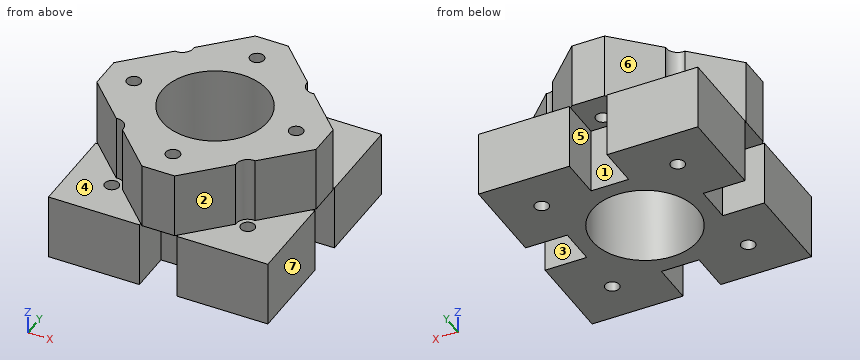
```python
from build123d import *

# Parameters (mm, degrees)
SKETCH_1_W          = 50
SKETCH_1_H          = 50
EXTRUDE_1_DEPTH     = 30
HOLE_WIZARD_348_D   = 24
HOLE_WIZARD_1_D     = 3.2
HOLE_WIZARD_2_D     = 3.2
CUT_EXTRUDE_1_DEPTH = 15
SKETCH_16_W         = 8.580132312
SKETCH_16_H         = 9.5
SKETCH_16_W_2       = 9.5
SKETCH_16_H_2       = 8.580132312
CUT_EXTRUDE_3_DEPTH = 15
HOLE_WIZARD_3_D     = 5.2
HOLE_WIZARD_3_DEPTH = 15


with BuildPart() as part:
    # 草图1 → 凸台-拉伸1 (new body)
    with BuildSketch(Plane.XY):
        Rectangle(SKETCH_1_W, SKETCH_1_H)
    extrude(amount=EXTRUDE_1_DEPTH)

    # Hole Wizard 348 (through all)
    with Locations(Plane.XY.offset(30)):
        with Locations((0, 0)):
            Hole(HOLE_WIZARD_348_D / 2)

    # 孔1 (through all)
    with Locations(Plane.XY.offset(30)):
        with Locations((-15.5, 15.5), (15.5, 15.5), (15.5, -15.5), (-15.5, -15.5)):
            Hole(HOLE_WIZARD_1_D / 2)

    # 孔2 (through all)
    with Locations(Plane.XY.offset(30)):
        with Locations((0, 18.5), (18.5, 0), (0, -18.5), (-18.5, 0)):
            Hole(HOLE_WIZARD_2_D / 2)

    # 草图13 → 切除-拉伸-薄壁1 (cut)
    with BuildSketch(Plane.XY.offset(30)):
        Polygon((-25, 3.7372583), (-14.36862915, 14.36862915), (-3.7372583, 25), (-17.879393924, 39.142135624), (-28.510764774, 28.510764774), (-39.142135624, 17.879393924), align=None)
        Polygon((3.7372583, 25), (14.36862915, 14.36862915), (25, 3.7372583), (39.142135624, 17.879393924), (28.510764774, 28.510764774), (17.879393924, 39.142135624), align=None)
        Polygon((-3.7372583, -25), (-14.36862915, -14.36862915), (-25, -3.7372583), (-39.142135624, -17.879393924), (-28.510764774, -28.510764774), (-17.879393924, -39.142135624), align=None)
        Polygon((25, -3.7372583), (14.36862915, -14.36862915), (3.7372583, -25), (17.879393924, -39.142135624), (28.510764774, -28.510764774), (39.142135624, -17.879393924), align=None)
    extrude(amount=-CUT_EXTRUDE_1_DEPTH, mode=Mode.SUBTRACT)

    # 草图16 → 切除-拉伸3 (cut)
    with BuildSketch(Plane(origin=(0, 0, 0), x_dir=(-1, 0, 0), z_dir=(0, 0, -1))):
        with Locations((0, 20.25)):
            Rectangle(SKETCH_16_W, SKETCH_16_H)
        with Locations((0, -20.25)):
            Rectangle(SKETCH_16_W, SKETCH_16_H)
        with Locations((-20.25, 0)):
            Rectangle(SKETCH_16_W_2, SKETCH_16_H_2)
        with Locations((20.25, 0)):
            Rectangle(SKETCH_16_W_2, SKETCH_16_H_2)
    extrude(amount=-CUT_EXTRUDE_3_DEPTH, mode=Mode.SUBTRACT)

    # 孔3
    with Locations(Plane.XY.offset(30)):
        with Locations((-15.5, 15.5), (15.5, 15.5), (15.5, -15.5), (-15.5, -15.5)):
            Hole(HOLE_WIZARD_3_D / 2, depth=HOLE_WIZARD_3_DEPTH)


solid = part.part
```
Check sheet for the modelled part. Datum: model origin and axes. Units: mm. Face numbers are marked on the shaded views. A direction names the side the tool comes from. Coordinates: 2 decimals unless noted, no trailing zeros. Order: outer loops, then holes, each group sorted by start corner. A loop starts at its lowest first (then second) coordinate and runs counter-clockwise, first axis right, second up. Notation, with made-up numbers: M -15,-32 L 14,-32 A37 ccw 14,7 Z; hole C 43,57 d1. An arc over 180 degrees is marked long. Write each question's results on one line, items separated by ' | '. Start each with the question number.
1. Access from +Z, -Z, +X, -X, +Y, -Y to the whole of each face (thin tool, end or side, straight path). Record for the marked faces 1, 2, 3 and 4.
2. Mould release check, pull along X, two halves, no side actions. Record for the marked faces 5, 6 and 7: +X half, -X half, draft (parallel to the pull), parting line (faces both ways), or undercut.
3. Material ranges on probe 1 along Y at (x, z) = (0, 26.25); probe 2 along X at (y, z) = (17.5, 6.25); probe 3 along Z at (x, y) = (22.5, -2.5), recorded low to high.
4. Cross-section at D-D on x = 18.5. Record the cut outline in (y, z).
5. Cross-section at A-A on x = 0. Record the cut outline in (y, z), and give its area (3 significant figures).
6. Cross-section at C-C on z = 9.25. Record the cut outline in (x, y), and give its area (3 significant figures).
7. Go/stop test with flat-tipped pins: P1, Ø9.5, axis at x = 20.5, y = -0.5, coming from the -Z side; P2, Ø5, axis at x = -15.5, y = -15.5, coming from the +Z side; P3, Ø6, axis at x = 0.5, y = 19.5, coming from the -Z side; P4, Ø1.5, axis at y = -3, z = 14, coming from the +X side. Record where each tip stops, or that it passes through.
Checks:
1) face 1: -Z, +Y | face 2: +Z, +X, -Y | face 3: -Z, +X | face 4: +Z, -X, -Y
2) face 5: undercut | face 6: -X half | face 7: +X half
3) probe 1: y = -25 to -20.1, -16.9 to -12, 12 to 16.9, 20.1 to 25 | probe 2: x = -25 to -4.29, 4.29 to 25 | probe 3: z = 15 to 30
4) outline: M -25,0 L -4.29,0 L -4.29,15 L -1.6,15 L -1.6,30 L -10.24,30 L -10.24,15 L -25,15 Z; M 1.6,15 L 4.29,15 L 4.29,0 L 25,0 L 25,15 L 10.24,15 L 10.24,30 L 1.6,30 Z
5) outline: M -25,15 L -20.1,15 L -20.1,30 L -25,30 Z; M -16.9,15 L -15.5,15 L -15.5,0 L -12,0 L -12,30 L -16.9,30 Z; M 12,0 L 15.5,0 L 15.5,15 L 16.9,15 L 16.9,30 L 12,30 Z; M 20.1,15 L 25,15 L 25,30 L 20.1,30 Z | area: 399 mm²
6) outline: M -25,-25 L -4.29,-25 L -4.29,-15.5 L 4.29,-15.5 L 4.29,-25 L 25,-25 L 25,-4.29 L 15.5,-4.29 L 15.5,4.29 L 25,4.29 L 25,25 L 4.29,25 L 4.29,15.5 L -4.29,15.5 L -4.29,25 L -25,25 L -25,4.29 L -15.5,4.29 L -15.5,-4.29 L -25,-4.29 Z; hole C -15.5,-15.5 d3.2; hole C -15.5,15.5 d3.2; hole C 0,0 d24; hole C 15.5,-15.5 d3.2; hole C 15.5,15.5 d3.2 | area: 1,690 mm²
7) P1: stops at z = 0 | P2: stops at z = 15 | P3: stops at z = 15 | P4: stops at x = 15.5
